```python
from build123d import *

# Parameters (mm, degrees)
SKETCH2_W           = 950
SKETCH2_H           = 440
BOSS_EXTRUDE1_DEPTH = 12.7
CUT_EXTRUDE1_REACH  = 525.628
SKETCH3_W           = 41
SKETCH3_H           = 41
CUT_EXTRUDE2_REACH  = 525.628
SKETCH4_R           = 2.75
CUT_EXTRUDE3_REACH  = 525.628
SKETCH6_R           = 2.665
CUT_EXTRUDE4_REACH  = 525.628
SKETCH7_R           = 2.665


with BuildPart() as part:
    # Sketch2 → Boss-Extrude1 (new body)
    with BuildSketch(Plane.XY):
        Rectangle(SKETCH2_W, SKETCH2_H)
    extrude(amount=BOSS_EXTRUDE1_DEPTH)

    # Sketch3 → Cut-Extrude1 (cut, up to next)
    with BuildSketch(Plane.XY.offset(12.7), mode=Mode.PRIVATE) as cut_extrude1_sk1:
        with Locations((-454.5, 199.5)):
            Rectangle(SKETCH3_W, SKETCH3_H)
    cut_extrude1_tool1 = extrude(cut_extrude1_sk1.sketch, amount=-CUT_EXTRUDE1_REACH, mode=Mode.PRIVATE) & part.part
    # Sketch3 → Cut-Extrude1 (cut, up to next)
    with BuildSketch(Plane.XY.offset(12.7), mode=Mode.PRIVATE) as cut_extrude1_sk2:
        with Locations((454.5, 199.5)):
            Rectangle(SKETCH3_W, SKETCH3_H)
    cut_extrude1_tool2 = extrude(cut_extrude1_sk2.sketch, amount=-CUT_EXTRUDE1_REACH, mode=Mode.PRIVATE) & part.part
    # Sketch3 → Cut-Extrude1 (cut, up to next)
    with BuildSketch(Plane.XY.offset(12.7), mode=Mode.PRIVATE) as cut_extrude1_sk3:
        with Locations((454.5, -199.5)):
            Rectangle(SKETCH3_W, SKETCH3_H)
    cut_extrude1_tool3 = extrude(cut_extrude1_sk3.sketch, amount=-CUT_EXTRUDE1_REACH, mode=Mode.PRIVATE) & part.part
    # Sketch3 → Cut-Extrude1 (cut, up to next)
    with BuildSketch(Plane.XY.offset(12.7), mode=Mode.PRIVATE) as cut_extrude1_sk4:
        with Locations((-454.5, -199.5)):
            Rectangle(SKETCH3_W, SKETCH3_H)
    cut_extrude1_tool4 = extrude(cut_extrude1_sk4.sketch, amount=-CUT_EXTRUDE1_REACH, mode=Mode.PRIVATE) & part.part
    add(cut_extrude1_tool1.solids().sort_by_distance((-454.5, 199.5, 12.7))[0], mode=Mode.SUBTRACT)
    add(cut_extrude1_tool2.solids().sort_by_distance((454.5, 199.5, 12.7))[0], mode=Mode.SUBTRACT)
    add(cut_extrude1_tool3.solids().sort_by_distance((454.5, -199.5, 12.7))[0], mode=Mode.SUBTRACT)
    add(cut_extrude1_tool4.solids().sort_by_distance((-454.5, -199.5, 12.7))[0], mode=Mode.SUBTRACT)

    # Sketch4 → Cut-Extrude2 (cut, up to next)
    with BuildSketch(Plane.XY.offset(12.7), mode=Mode.PRIVATE) as cut_extrude2_sk1:
        with Locations((-465, -154)):
            Circle(SKETCH4_R)
    cut_extrude2_tool1 = extrude(cut_extrude2_sk1.sketch, amount=-CUT_EXTRUDE2_REACH, mode=Mode.PRIVATE) & part.part
    # Sketch4 → Cut-Extrude2 (cut, up to next)
    with BuildSketch(Plane.XY.offset(12.7), mode=Mode.PRIVATE) as cut_extrude2_sk2:
        with Locations(Location((-465, 154, 0), (0, 0, 180))):
            Circle(SKETCH4_R)
    cut_extrude2_tool2 = extrude(cut_extrude2_sk2.sketch, amount=-CUT_EXTRUDE2_REACH, mode=Mode.PRIVATE) & part.part
    # Sketch4 → Cut-Extrude2 (cut, up to next)
    with BuildSketch(Plane.XY.offset(12.7), mode=Mode.PRIVATE) as cut_extrude2_sk3:
        with Locations(Location((465, -154, 0), (0, 0, 180))):
            Circle(SKETCH4_R)
    cut_extrude2_tool3 = extrude(cut_extrude2_sk3.sketch, amount=-CUT_EXTRUDE2_REACH, mode=Mode.PRIVATE) & part.part
    # Sketch4 → Cut-Extrude2 (cut, up to next)
    with BuildSketch(Plane.XY.offset(12.7), mode=Mode.PRIVATE) as cut_extrude2_sk4:
        with Locations((465, 154)):
            Circle(SKETCH4_R)
    cut_extrude2_tool4 = extrude(cut_extrude2_sk4.sketch, amount=-CUT_EXTRUDE2_REACH, mode=Mode.PRIVATE) & part.part
    add(cut_extrude2_tool1.solids().sort_by_distance((-465, -154, 12.7))[0], mode=Mode.SUBTRACT)
    add(cut_extrude2_tool2.solids().sort_by_distance((-465, 154, 12.7))[0], mode=Mode.SUBTRACT)
    add(cut_extrude2_tool3.solids().sort_by_distance((465, -154, 12.7))[0], mode=Mode.SUBTRACT)
    add(cut_extrude2_tool4.solids().sort_by_distance((465, 154, 12.7))[0], mode=Mode.SUBTRACT)

    # Sketch6 → Cut-Extrude3 (cut, up to next)
    with BuildSketch(Plane.XY.offset(12.7), mode=Mode.PRIVATE) as cut_extrude3_sk1:
        with Locations((-153.985226099, -167.605059616)):
            Circle(SKETCH6_R)
    cut_extrude3_tool1 = extrude(cut_extrude3_sk1.sketch, amount=-CUT_EXTRUDE3_REACH, mode=Mode.PRIVATE) & part.part
    # Sketch6 → Cut-Extrude3 (cut, up to next)
    with BuildSketch(Plane.XY.offset(12.7), mode=Mode.PRIVATE) as cut_extrude3_sk2:
        with Locations((214.314773901, -167.605059616)):
            Circle(SKETCH6_R)
    cut_extrude3_tool2 = extrude(cut_extrude3_sk2.sketch, amount=-CUT_EXTRUDE3_REACH, mode=Mode.PRIVATE) & part.part
    # Sketch6 → Cut-Extrude3 (cut, up to next)
    with BuildSketch(Plane.XY.offset(12.7), mode=Mode.PRIVATE) as cut_extrude3_sk3:
        with Locations((214.314773901, 162.594940384)):
            Circle(SKETCH6_R)
    cut_extrude3_tool3 = extrude(cut_extrude3_sk3.sketch, amount=-CUT_EXTRUDE3_REACH, mode=Mode.PRIVATE) & part.part
    # Sketch6 → Cut-Extrude3 (cut, up to next)
    with BuildSketch(Plane.XY.offset(12.7), mode=Mode.PRIVATE) as cut_extrude3_sk4:
        with Locations((-153.985226099, 162.594940384)):
            Circle(SKETCH6_R)
    cut_extrude3_tool4 = extrude(cut_extrude3_sk4.sketch, amount=-CUT_EXTRUDE3_REACH, mode=Mode.PRIVATE) & part.part
    add(cut_extrude3_tool1.solids().sort_by_distance((-153.985226, -167.60506, 12.7))[0], mode=Mode.SUBTRACT)
    add(cut_extrude3_tool2.solids().sort_by_distance((214.314774, -167.60506, 12.7))[0], mode=Mode.SUBTRACT)
    add(cut_extrude3_tool3.solids().sort_by_distance((214.314774, 162.59494, 12.7))[0], mode=Mode.SUBTRACT)
    add(cut_extrude3_tool4.solids().sort_by_distance((-153.985226, 162.59494, 12.7))[0], mode=Mode.SUBTRACT)

    # Sketch7 → Cut-Extrude4 (cut, up to next)
    with BuildSketch(Plane.XY.offset(12.7), mode=Mode.PRIVATE) as cut_extrude4_sk1:
        with Locations((429, 4)):
            Circle(SKETCH7_R)
    cut_extrude4_tool1 = extrude(cut_extrude4_sk1.sketch, amount=-CUT_EXTRUDE4_REACH, mode=Mode.PRIVATE) & part.part
    # Sketch7 → Cut-Extrude4 (cut, up to next)
    with BuildSketch(Plane.XY.offset(12.7), mode=Mode.PRIVATE) as cut_extrude4_sk2:
        with Locations((429, -154)):
            Circle(SKETCH7_R)
    cut_extrude4_tool2 = extrude(cut_extrude4_sk2.sketch, amount=-CUT_EXTRUDE4_REACH, mode=Mode.PRIVATE) & part.part
    # Sketch7 → Cut-Extrude4 (cut, up to next)
    with BuildSketch(Plane.XY.offset(12.7), mode=Mode.PRIVATE) as cut_extrude4_sk3:
        with Locations((316, 4)):
            Circle(SKETCH7_R)
    cut_extrude4_tool3 = extrude(cut_extrude4_sk3.sketch, amount=-CUT_EXTRUDE4_REACH, mode=Mode.PRIVATE) & part.part
    # Sketch7 → Cut-Extrude4 (cut, up to next)
    with BuildSketch(Plane.XY.offset(12.7), mode=Mode.PRIVATE) as cut_extrude4_sk4:
        with Locations((316, -154)):
            Circle(SKETCH7_R)
    cut_extrude4_tool4 = extrude(cut_extrude4_sk4.sketch, amount=-CUT_EXTRUDE4_REACH, mode=Mode.PRIVATE) & part.part
    add(cut_extrude4_tool1.solids().sort_by_distance((429, 4, 12.7))[0], mode=Mode.SUBTRACT)
    add(cut_extrude4_tool2.solids().sort_by_distance((429, -154, 12.7))[0], mode=Mode.SUBTRACT)
    add(cut_extrude4_tool3.solids().sort_by_distance((316, 4, 12.7))[0], mode=Mode.SUBTRACT)
    add(cut_extrude4_tool4.solids().sort_by_distance((316, -154, 12.7))[0], mode=Mode.SUBTRACT)


solid = part.part
```
Input: part model. Units: mm. Frame: model coordinates. Give positions to 0.01 mm unless a question says otherwise; leave off trailing zeros. Return JSON: item names as keys, results as strings.
1) Line query: L1, parallel to Y at x = 429, z = 9 (3 decimals); L2, parallel to X at y = -154, z = 4 (3 decimals); L3, parallel to Y at x = 465, z = 9.75. Output: solid intervals per line, ascending. Write a range as [from, to].
Taken from the geometry:
{"L1": "y = [-220, -156.665], [-151.335, 1.335], [6.665, 220]", "L2": "x = [-475, -467.75], [-462.25, 313.335], [318.665, 426.335], [431.665, 462.25], [467.75, 475]", "L3": "y = [-179, -156.75], [-151.25, 151.25], [156.75, 179]"}
2) Section query A-A on z = 3. Count the separate pieces of the cut face and the enclosed holes in it, and give its area (3 significant figures).
Taken from the geometry:
{"separate pieces": "1", "enclosed holes": "12", "area": "411,000 mm2"}
3) Contact query for flat-ended pins moving along their axis: pin 1 (5 mm diameter, centred on x = -153.99, y = -167.61, fed in from +Z); pin 2 (6.5 mm diameter, centred on y = -200.5, z = 6.5, fed in from -X). Output: stop coordinate, or through.
Taken from the geometry:
{"pin 1": "passes through", "pin 2": "stops at x = -434"}
